Geometry: final body of the model. Coordinates: model frame, mm. Round coordinates to 2 decimals unless told otherwise and drop trailing zeros. Loops run counter-clockwise (first coordinate to the right, second up) from the corner with the lowest first, then second, coordinate; pieces in that order, holes last. Notation, with made-up numbers: (27.5, -30) - (56.5, -30) arc R22 ccw to (56.5, -6) - close; hole circle Ø8 at (73.5, -31). An arc over 180 degrees is marked (long way). Return JSON: item names as keys, results as strings. Group by question number.
1. Material intervals for probe 1 along Z at (x, y) = (-67.5, 0.6); probe 2 along X at (y, z) = (1.5, 3); probe 3 along Z at (x, y) = (67.5, 1.8), sorted ascending.
2. Section A-A on z = 0. Return loops of the section in (x, y).
3. Section C-C on y = 2.9. Return loops of the section in (x, z), and give its area (3 significant figures).
4. Draft query along Z for faces 1 (the face through (1, 4, 0)), 2 (the face through (-66, 0.9, -4)), 3 (the face through (74, 2, 0)), 4 (the face through (-71.27, 0.44, -2.89)). Return one class per face: +Z half, -Z half, draft (parallel to the pull), parting line (faces both ways), or undercut.
5. Section B-B on x = -65. Return loops of the section in (y, z).
from build123d import *

# Parameters (mm, degrees)
EXTRUDE_1_DEPTH              = 4
HOLE_WIZARD_M5_1_D           = 8
HOLE_WIZARD_M5_1_DEPTH       = 12.4
HOLE_WIZARD_M5_1_CBORE_D     = 9.5
HOLE_WIZARD_M5_1_CBORE_DEPTH = 0.9
HOLE_WIZARD_M5_1_TIP         = 2.403442476
HOLE_WIZARD_M3_1_D           = 3
HOLE_WIZARD_M3_1_DEPTH       = 7.5
HOLE_WIZARD_M3_1_TIP         = 0.901290929


with BuildPart() as part:
    # 草图1 → 凸台-拉伸1 (new body)
    with BuildSketch(Plane(origin=(0, 0, 0), x_dir=(1, 0, 0), z_dir=(0, 1, 0))):
        with BuildLine():
            Line((-67.5, 6.5), (67.5, 6.5))
            ThreePointArc((67.5, 6.5), (74, 0), (67.5, -6.5))
            Line((67.5, -6.5), (-67.5, -6.5))
            ThreePointArc((-67.5, -6.5), (-74, 0), (-67.5, 6.5))
        make_face()
    extrude(amount=EXTRUDE_1_DEPTH)

    # M5 六角头螺栓的柱形沉头孔1
    with Locations(Plane.XZ):
        with Locations((-67.5, 0)):
            CounterBoreHole(HOLE_WIZARD_M5_1_D / 2, HOLE_WIZARD_M5_1_CBORE_D / 2, HOLE_WIZARD_M5_1_CBORE_DEPTH, depth=HOLE_WIZARD_M5_1_DEPTH)
            with Locations((0, 0, -(HOLE_WIZARD_M5_1_DEPTH + HOLE_WIZARD_M5_1_TIP / 2))):  # 118° drill point
                Cone(0, HOLE_WIZARD_M5_1_D / 2, HOLE_WIZARD_M5_1_TIP, mode=Mode.SUBTRACT)

    # M3 螺纹孔1
    with Locations(Plane(origin=(0, 4, 0), x_dir=(1, 0, 0), z_dir=(0, 1, 0))):
        with Locations((67.5, 0)):
            Hole(HOLE_WIZARD_M3_1_D / 2, depth=HOLE_WIZARD_M3_1_DEPTH)
            with Locations((0, 0, -(HOLE_WIZARD_M3_1_DEPTH + HOLE_WIZARD_M3_1_TIP / 2))):  # 118° drill point
                Cone(0, HOLE_WIZARD_M3_1_D / 2, HOLE_WIZARD_M3_1_TIP, mode=Mode.SUBTRACT)


solid = part.part
Taken from the geometry:
{
 "1": {"probe 1": "-6.5 to -4.75, 4.75 to 6.5", "probe 2": "-73.27 to -70.15, -64.85 to 73.27", "probe 3": "-6.5 to -1.5, 1.5 to 6.5"},
 "2": {"outline": "(-74, 0) - (-72.25, 0) - (-72.25, 0.9) - (-71.5, 0.9) - (-71.5, 4) - (-74, 4) - close; (-63.5, 0.9) - (-62.75, 0.9) - (-62.75, 0) - (66, 0) - (66, 4) - (-63.5, 4) - close; (69, 0) - (74, 0) - (74, 4) - (69, 4) - close"},
 "3": {"outline": "(-67.5, -6.5) - (67.5, -6.5) arc R6.5 ccw to (67.5, 6.5) - (-67.5, 6.5) arc R6.5 ccw to start; hole circle Ø8 at (-67.5, 0); hole circle Ø3 at (67.5, 0)", "area": "1,830 mm2"},
 "4": {"face 1": "draft", "face 2": "undercut", "face 3": "parting line", "face 4": "undercut"},
 "5": {"outline": "(0, -6.5) - (4, -6.5) - (4, -3.12) - (0.9, -3.12) - (0.9, -4.04) - (0, -4.04) - close; (0, 4.04) - (0.9, 4.04) - (0.9, 3.12) - (4, 3.12) - (4, 6.5) - (0, 6.5) - close"}
}
